from build123d import *

# Parameters (mm, degrees)
F0_W     = 55.832479
F0_H     = 49.21193
F1_DEPTH = 61.468
F2_SIZE  = 5.08
F3_SIZE  = 5.08


with BuildPart() as f1:
    # F0 (on Front) → F1 (new body)
    with BuildSketch(Plane.XZ):
        with Locations((-27.916239, 24.605965)):
            Rectangle(F0_W, F0_H)
    extrude(amount=F1_DEPTH)

    # F2
    f2_edges = [f1.edges().sort_by_distance(p)[0] for p in [
        (0, -30.734, 49.21193),
        (-27.91624, -61.468, 49.21193),
        (-55.832479, -30.734, 49.21193),
        (-27.91624, 0, 49.21193),
    ]]
    chamfer(f2_edges, length=F2_SIZE)

    # F3
    f3_edges = [f1.edges().sort_by_distance(p)[0] for p in [
        (0, -30.734, 0),
        (-27.91624, -61.468, 0),
        (-55.832479, -30.734, 0),
        (-27.91624, 0, 0),
    ]]
    chamfer(f3_edges, length=F3_SIZE)


solid = f1.part
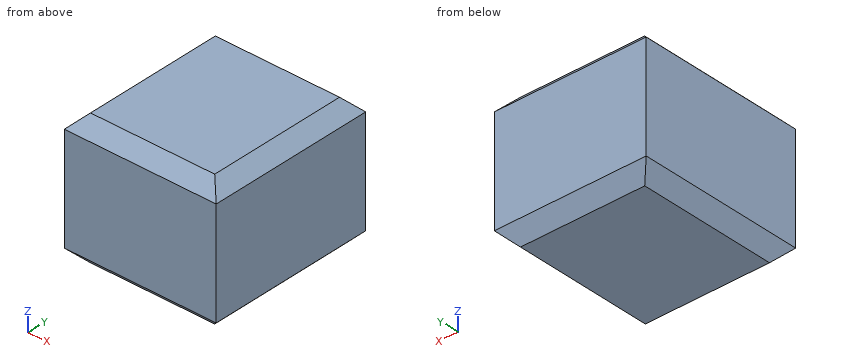
The model under review builds one solid part; all positions refer to its coordinate system, in mm. Give positions to 0.01 mm unless a question says otherwise; leave off trailing zeros. Loops run counter-clockwise (first coordinate to the right, second up) from the corner with the lowest first, then second, coordinate; pieces in that order, holes last. Notation, with made-up numbers: (5, 39.25) -> (36, 39.25) arc R33 cw to (36, 78.25) -> close; hole circle Ø9 at (-6.75, 77). An arc over 180 degrees is marked (long way). Answer as a JSON object with one key per item and string values. Group by question number.
Q1. Wall thickness on line 1 along Y through (x, z) = (-18, 3.5); line 2 along X through (y, z) = (-21, 3); line 3 along Z through (x, y) = (-16, -4): over which ranges is each line inside the solid? List them lowest first.
Q2. Take a section at B-B (x = -39). Write out the cut boundary in (y, z).
Q3. Take a section at A-A (y = -45). Write out the cut boundary in (x, z), plus the area to 3 significant figures.
Q4. Take a section at D-D (z = 46). Write out the cut boundary in (x, y).
Q5. Insertion check: pin 1 (1.5 mm diameter, centred on x = -49, z = 40.5, fed in from +Y). The pin has a flat end and moves straight along its axis. Give the tip position at first contact, or say it passes through.
Q6. Take a section at C-C (z = 3.5). Write out the cut boundary in (x, y), plus the area to 3 significant figures.
Answer below:
{
 "1": {"line 1": "y = -59.89 to -1.58", "line 2": "x = -53.75 to -2.08", "line 3": "z = 1.08 to 48.13"},
 "2": {"outline": "(-61.47, 5.08) -> (-56.39, 0) -> (-5.08, 0) -> (0, 5.08) -> (0, 44.13) -> (-5.08, 49.21) -> (-56.39, 49.21) -> (-61.47, 44.13) -> close"},
 "3": {"outline": "(-55.83, 5.08) -> (-50.75, 0) -> (-5.08, 0) -> (0, 5.08) -> (0, 44.13) -> (-5.08, 49.21) -> (-50.75, 49.21) -> (-55.83, 44.13) -> close", "area": "2,700 mm2"},
 "4": {"outline": "(-53.96, -59.6) -> (-1.87, -59.6) -> (-1.87, -1.87) -> (-53.96, -1.87) -> close"},
 "5": {"pin 1": "stops at y = 0"},
 "6": {"outline": "(-54.25, -59.89) -> (-1.58, -59.89) -> (-1.58, -1.58) -> (-54.25, -1.58) -> close", "area": "3,070 mm2"}
}
